Geometry check sheet. Reference: the model listing, model coordinates, mm. A direction names the side the tool comes from. Coordinates: 2 decimals unless noted, no trailing zeros. Loops run counter-clockwise (first coordinate to the right, second up) from the corner with the lowest first, then second, coordinate; pieces in that order, holes last.
from build123d import *

# Parameters (mm, degrees)
SKETCH_1_W      = 22.5
SKETCH_1_H      = 12.5
EXTRUDE_1_DEPTH = 16
EXTRUDE_2_DEPTH = 2
SKETCH_3_W      = 22.5
SKETCH_3_H      = 12.5
EXTRUDE_3_DEPTH = 4.7
SKETCH_4_R      = 5
EXTRUDE_4_DEPTH = 3
SKETCH_5_R      = 2
EXTRUDE_5_DEPTH = 5


with BuildPart() as part:
    # 草图1 → 凸台-拉伸1 (new body)
    with BuildSketch(Plane(origin=(0, 0, 0), x_dir=(1, 0, 0), z_dir=(0, 1, 0))):
        Rectangle(SKETCH_1_W, SKETCH_1_H)
    extrude(amount=EXTRUDE_1_DEPTH)

    # 草图2 → 凸台-拉伸2 (add)
    with BuildSketch(Plane(origin=(0, 16, 0), x_dir=(1, 0, 0), z_dir=(0, 1, 0))):
        with BuildLine():
            Line((-15.9, 6.25), (15.9, 6.25))
            Line((15.9, 6.25), (15.9, 0.5))
            Line((15.9, 0.5), (14.979795897, 0.5))
            ThreePointArc((14.979795897, 0.5), (12.9, 0), (14.979795897, -0.5))
            Line((14.979795897, -0.5), (15.9, -0.5))
            Line((15.9, -0.5), (15.9, -6.25))
            Line((15.9, -6.25), (-15.9, -6.25))
            Line((-15.9, -6.25), (-15.9, -0.5))
            Line((-15.9, -0.5), (-14.979795897, -0.5))
            ThreePointArc((-14.979795897, -0.5), (-12.9, 0), (-14.979795897, 0.5))
            Line((-14.979795897, 0.5), (-15.9, 0.5))
            Line((-15.9, 0.5), (-15.9, 6.25))
        make_face()
    extrude(amount=EXTRUDE_2_DEPTH)

    # 草图3 → 凸台-拉伸3 (add)
    with BuildSketch(Plane(origin=(0, 18, 0), x_dir=(1, 0, 0), z_dir=(0, 1, 0))):
        Rectangle(SKETCH_3_W, SKETCH_3_H)
    extrude(amount=EXTRUDE_3_DEPTH)

    # 草图4 → 凸台-拉伸4 (add)
    with BuildSketch(Plane(origin=(0, 22.7, 0), x_dir=(1, 0, 0), z_dir=(0, 1, 0))):
        with Locations((6.25, 0)):
            Circle(SKETCH_4_R)
    extrude(amount=EXTRUDE_4_DEPTH)

    # 草图5 → 凸台-拉伸5 (add)
    with BuildSketch(Plane(origin=(0, 25.7, 0), x_dir=(1, 0, 0), z_dir=(0, 1, 0))):
        with Locations(Location((6.25, 0, 0), (0, 0, 270))):
            Circle(SKETCH_5_R)
    extrude(amount=EXTRUDE_5_DEPTH)


solid = part.part
1) Material ranges on probe 1 along Z at (x, y) = (14, 17); probe 2 along Y at (x, z) = (-11.5, -2.5); probe 3 along X at (y, z) = (3, -2), recorded low to high.
Data:
probe 1: z = -6.25 to -1.1, 1.1 to 6.25
probe 2: y = 16 to 18
probe 3: x = -11.25 to 11.25
2) Section check B-B on x = 6.25. Record the cut outline in (y, z).
Data:
outline: (0, -6.25) - (22.7, -6.25) - (22.7, -5) - (25.7, -5) - (25.7, -2) - (30.7, -2) - (30.7, 2) - (25.7, 2) - (25.7, 5) - (22.7, 5) - (22.7, 6.25) - (0, 6.25) - close
3) Mould release check, pull along X, two halves, no side actions. Record for faces 6 (the cylindrical face through (12.9, 17, 0)), 7 (the flat face through (15.4, 17, -0.5)), 8 (the cylindrical face through (-12.9, 17, 0)), 9 (the flat face through (15.9, 17, -3)): +X half, -X half, draft (parallel to the pull), parting line (faces both ways), or undercut.
Data:
face 6: undercut
face 7: draft
face 8: undercut
face 9: +X half
4) Section check D-D on y = 29. Record the cut outline in (x, z), and give its area (3 significant figures).
Data:
outline: circle Ø4 at (6.25, 0)
area: 12.6 mm2
5) Access from +Z, -Z, +X, -X, +Y, -Y to the whole of each face (thin tool, end or side, straight path). Record for faces 1 (the flat face through (15.4, 17, 0.5)), 2 (the flat face through (11.25, 8, 0)), 3 (the cylindrical face through (8.233, 28.165, -0.26)), 4 (the flat face through (11.25, 20, 0)), 5 (the flat face through (-11.25, 8, 0)).
Data:
face 1: +X, +Y, -Y
face 2: +Z, -Z, +X, -Y
face 3: +Y
face 4: +Z, -Z, +X, +Y
face 5: +Z, -Z, -X, -Y
6) Section check A-A on x = -14. Record the cut outline in (y, z), and give its area (3 significant figures).
Data:
outline: (16, -6.25) - (18, -6.25) - (18, -1.1) - (16, -1.1) - close; (16, 1.1) - (18, 1.1) - (18, 6.25) - (16, 6.25) - close
area: 20.6 mm2
7) Section check C-C on z = 4. Record the cut outline in (x, y).
Data:
outline: (-15.9, 16) - (-11.25, 16) - (-11.25, 0) - (11.25, 0) - (11.25, 16) - (15.9, 16) - (15.9, 18) - (11.25, 18) - (11.25, 22.7) - (9.25, 22.7) - (9.25, 25.7) - (3.25, 25.7) - (3.25, 22.7) - (-11.25, 22.7) - (-11.25, 18) - (-15.9, 18) - close
8) Depth check by flat-ended pin: pin 1 (3 mm diameter, centred on x = -14, z = 0, fed in from -Y); pin 2 (5 mm diameter, centred on y = 9, z = -0.5, fed in from +X); pin 3 (1.5 mm diameter, centred on y = 11.5, z = 2, fed in from -X); pin 4 (1.8 mm diameter, centred on x = 14, z = 0, fed in from +Y). Enter the tip coordinate at first touch or a pass-through.
Data:
pin 1: stops at y = 16
pin 2: stops at x = 11.25
pin 3: stops at x = -11.25
pin 4: passes through
